Verification items for the finished model (mm, model axes). Face numbers are marked on the shaded views. Give positions to 0.01 mm unless a question says otherwise; leave off trailing zeros. Order: outer loops, then holes, each group sorted by start corner. A loop starts at its lowest first (then second) coordinate and runs counter-clockwise, first axis right, second up. Notation, with made-up numbers: (85, 23.25) -> (144, 23.25) arc R26 cw to (144, 61.25) -> close; hole circle Ø6 at (28, 36). An arc over 180 degrees is marked (long way). Write each question's results on one line, items separated by ' | '. Start each with the question number.
1. Cross-section at B-B, the plane x = -82. Enter the section's corners in (y, z).
2. Cross-section at D-D, the plane x = -9. Enter the section's corners in (y, z).
3. Material ranges on L1, parallel to X at y = -30.5, z = 96; L2, parallel to Z at x = -61, y = 1.5; L3, parallel to Z at x = -74, y = -2, recorded low to high. Write a range as from..to.
4. Depth check by flat-ended pin: pin 1 Ø19 at (y, z) = (-22.5, 289) entering from +X; pin 2 Ø3 at (x, z) = (-10, 90) entering from +Y; pin 3 Ø10 at (x, y) = (-79, -1.5) entering from -Z. Enter the tip coordinate at first touch or a pass-through.
5. Cross-section at A-A, the plane z = 190. Enter the section's corners in (x, y).
6. Cross-section at C-C, the plane y = -28. Enter the section's corners in (x, z).
7. Mould release check, pull along X, two halves, no side actions. Record for the marked faces 1, 2 and 3: +X half, -X half, draft (parallel to the pull), parting line (faces both ways), or undercut.
from build123d import *

# Parameters (mm, degrees)
BOSS_EXTRUDE1_DEPTH = 406.4
SKETCH4_W           = 73.282534648
SKETCH4_H           = 7.62
BOSS_EXTRUDE4_DEPTH = 10.16
BOSS_EXTRUDE5_START = -7.62
SKETCH7_W           = 25.022534648
SKETCH7_H           = 36.83
BOSS_EXTRUDE5_DEPTH = 7.62
BOSS_EXTRUDE6_START = -7.62
SKETCH11_W          = 25.022534648
SKETCH11_H          = 36.83
BOSS_EXTRUDE6_DEPTH = 7.62
BOSS_EXTRUDE7_DEPTH = 12.7
CHAMFER3_SIZE       = 1.905
CHAMFER4_SIZE       = 5.08
CHAMFER4_SIZE2      = 1.361181898


with BuildPart() as part:
    # Sketch1 → Boss-Extrude1 (new body)
    with BuildSketch(Plane.XY):
        Polygon((-36.83, -4.9276), (7.62, -4.9276), (7.62, 0), (0, 0), (0, -2.3876), (-29.21, -2.3876), (-40.64, -2.3876), (-40.64, -39.2176), (-65.662534648, -39.2176), (-65.662534648, 7.7724), (-69.472534648, 7.7724), (-69.472534648, -43.0276), (-36.83, -43.0276), align=None)
    extrude(amount=BOSS_EXTRUDE1_DEPTH)

    # Sketch4 → Boss-Extrude4 (add)
    with BuildSketch(Plane(origin=(0, -2.3876, 0), x_dir=(1, 0, 0), z_dir=(0, 1, 0))):
        with Locations((-29.021267324, -402.59)):
            Rectangle(SKETCH4_W, SKETCH4_H)
        with Locations((-29.021267324, -3.81)):
            Rectangle(SKETCH4_W, SKETCH4_H)
    extrude(amount=BOSS_EXTRUDE4_DEPTH)

    # Sketch7 → Boss-Extrude5 (add)
    with BuildSketch(Plane.XY.offset(406.4).offset(BOSS_EXTRUDE5_START)):
        with Locations((-53.151267324, -20.8026)):
            Rectangle(SKETCH7_W, SKETCH7_H)
    extrude(amount=BOSS_EXTRUDE5_DEPTH)

    # Sketch11 → Boss-Extrude6 (add)
    with BuildSketch(Plane(origin=(0, 0, 0), x_dir=(-1, 0, 0), z_dir=(0, 0, -1)).offset(BOSS_EXTRUDE6_START)):
        with Locations((53.151267324, -20.8026)):
            Rectangle(SKETCH11_W, SKETCH11_H)
    extrude(amount=BOSS_EXTRUDE6_DEPTH)

    # Sketch15 → Boss-Extrude7 (add)
    with BuildSketch(Plane(origin=(0, 7.7724, 0), x_dir=(1, 0, 0), z_dir=(0, 1, 0))):
        Polygon((-69.472534648, -256.308132937), (-69.472534648, -249.958132937), (-88.522534648, -249.958132937), (-88.522534648, -148.358132937), (-69.472534648, -148.358132937), (-69.472534648, -142.008132937), (-94.872534648, -142.008132937), (-94.872534648, -256.308132937), align=None)
    extrude(amount=-BOSS_EXTRUDE7_DEPTH)

    # Chamfer3
    chamfer3_edges = [part.edges().sort_by_distance(p)[0] for p in [
        (-88.522534648, -4.9276, 199.158132937),
        (-94.872534648, -4.9276, 199.158132937),
        (-94.872534648, 7.7724, 199.158132937),
        (-88.522534648, 7.7724, 199.158132937),
    ]]
    chamfer(chamfer3_edges, length=CHAMFER3_SIZE)

    # Chamfer4
    chamfer4_edges = [part.edges().sort_by_distance(p)[0] for p in [
        (0, 0, 203.2),
    ]]
    chamfer4_side = [part.faces().sort_by_distance(p)[0] for p in [
        (3.81, 0, 203.2),
    ]]
    chamfer(chamfer4_edges, length=CHAMFER4_SIZE, length2=CHAMFER4_SIZE2, reference=chamfer4_side[0])


solid = part.part
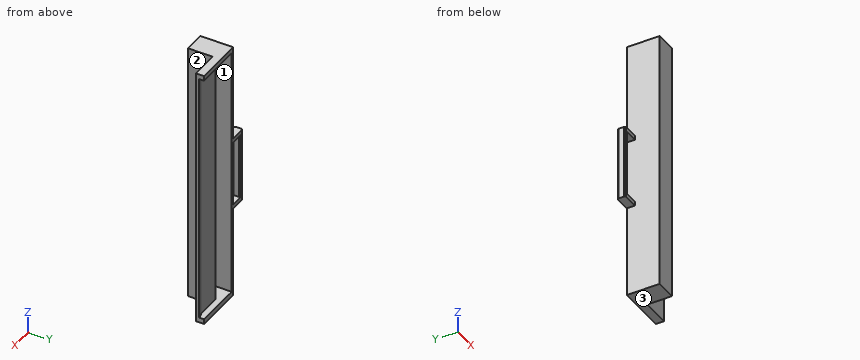
Results below:
1) outline: (-4.93, 142.01) -> (7.77, 142.01) -> (7.77, 148.36) -> (-4.93, 148.36) -> close; (-4.93, 249.96) -> (7.77, 249.96) -> (7.77, 256.31) -> (-4.93, 256.31) -> close
2) outline: (-4.93, 0) -> (7.77, 0) -> (7.77, 7.62) -> (-2.39, 7.62) -> (-2.39, 398.78) -> (7.77, 398.78) -> (7.77, 406.4) -> (-4.93, 406.4) -> close
3) L1: x = -69.47..-65.66, -40.64..-36.83 | L2: z = 0..7.62, 398.78..406.4 | L3: z = 142.01..148.36, 249.96..256.31
4) pin 1: stops at x = -36.83 | pin 2: stops at y = -2.39 | pin 3: stops at z = 142.01
5) outline: (-94.87, -3.02) -> (-92.97, -4.93) -> (-90.43, -4.93) -> (-88.52, -3.02) -> (-88.52, 5.87) -> (-90.43, 7.77) -> (-92.97, 7.77) -> (-94.87, 5.87) -> close; (-69.47, -43.03) -> (-36.83, -43.03) -> (-36.83, -4.93) -> (7.62, -4.93) -> (7.62, 0) -> (5.08, 0) -> (0, -1.36) -> (0, -2.39) -> (-40.64, -2.39) -> (-40.64, -39.22) -> (-65.66, -39.22) -> (-65.66, 7.77) -> (-69.47, 7.77) -> close
6) outline: (-69.47, 0) -> (-36.83, 0) -> (-36.83, 406.4) -> (-69.47, 406.4) -> close; hole (-65.66, 7.62) -> (-40.64, 7.62) -> (-40.64, 398.78) -> (-65.66, 398.78) -> close
7) face 1: undercut | face 2: +X half | face 3: draft
